```python
from build123d import *

# Parameters (mm, degrees)
SKETCH1_W                = 14.986
SKETCH1_H                = 10.16
BOSS_EXTRUDE1_DEPTH      = 3.175
M3_CLEARANCE_HOLE1_D     = 3.4
M3_CLEARANCE_HOLE1_DEPTH = 10
M3_CLEARANCE_HOLE1_TIP   = 1.021463052
SKETCH4_R                = 0.396875
CUT_EXTRUDE1_DEPTH       = 19.38168711


with BuildPart() as part:
    # Sketch1 → Boss-Extrude1 (new body)
    with BuildSketch(Plane.XY):
        with Locations((7.493, 5.08)):
            Rectangle(SKETCH1_W, SKETCH1_H)
    extrude(amount=BOSS_EXTRUDE1_DEPTH)

    # M3 Clearance Hole1
    with Locations(Plane.XY.offset(3.175)):
        with Locations((10.9982, 5.08), (3.9878, 5.08)):
            Hole(M3_CLEARANCE_HOLE1_D / 2, depth=M3_CLEARANCE_HOLE1_DEPTH)
            with Locations((0, 0, -(M3_CLEARANCE_HOLE1_DEPTH + M3_CLEARANCE_HOLE1_TIP / 2))):  # 118° drill point
                Cone(0, M3_CLEARANCE_HOLE1_D / 2, M3_CLEARANCE_HOLE1_TIP, mode=Mode.SUBTRACT)

    # Sketch4 → Cut-Extrude1 (cut, through all)
    with BuildSketch(Plane.XY.offset(3.175)):
        with Locations((7.493, 5.08)):
            Circle(SKETCH4_R)
    extrude(amount=-CUT_EXTRUDE1_DEPTH, mode=Mode.SUBTRACT)


solid = part.part
```
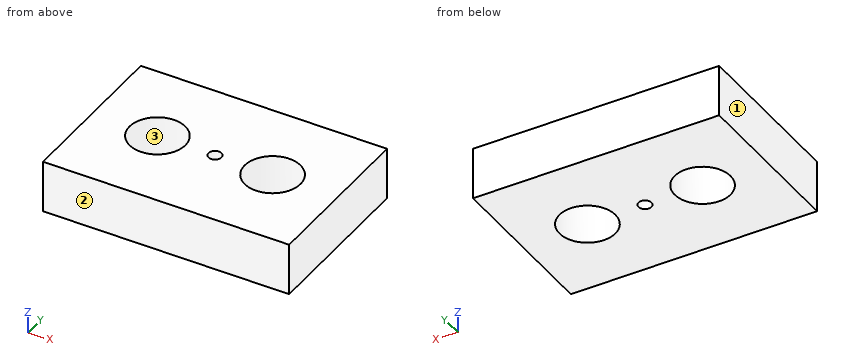
The model under review builds one solid part; all positions refer to its coordinate system, in mm. Face numbers are marked on the shaded views. Give positions to 0.01 mm unless a question says otherwise; leave off trailing zeros. Write each loop counter-clockwise with the first axis right and the second up, starting at its lowest first coordinate (ties: lowest second). Pieces come first, ordered by that corner, then holes. Notation, with made-up numbers: (11, 77.25) - (35, 77.25) arc R22 ccw to (35, 97.25) - close; hole circle Ø11 at (72, -5). An arc over 180 degrees is marked (long way). Answer in a Markdown table with one row per item. Add a question column.
1. We need section A-A on y = 5.08. Write out the cut boundary in (x, z) (3 decimals).
2. Draft analysis for pull direction X (two halves, no side actions). For the marked faces 1, 2 and 3, state which applies: +X half, -X half, draft (parallel to the pull), parting line (faces both ways), or undercut.
3. Wall thickness on line 1 along X through (y, z) = (4.75, 2.3); line 2 along Y through (x, z) = (7.5, 2.8); line 3 along X through (y, z) = (4, 0.55): over which ranges is each line inside the solid? List them lowest first. Write a range as [from, to].
4. We need section B-B on x = 9.5. Write out the cut boundary in (y, z) (3 decimals).
5. We need section C-C on z = 0.7. Write out the cut boundary in (x, y).
Ans:
| question | item | result |
|---|---|---|
| 1 | outline | (0, 0) - (2.288, 0) - (2.288, 3.175) - (0, 3.175) - close; (5.688, 0) - (7.096, 0) - (7.096, 3.175) - (5.688, 3.175) - close; (7.89, 0) - (9.298, 0) - (9.298, 3.175) - (7.89, 3.175) - close; (12.698, 0) - (14.986, 0) - (14.986, 3.175) - (12.698, 3.175) - close |
| 2 | face 1 | -X half |
| 2 | face 2 | draft |
| 2 | face 3 | undercut |
| 3 | line 1 | x = [0, 2.32], [5.66, 7.27], [7.71, 9.33], [12.67, 14.99] |
| 3 | line 2 | y = [0, 4.68], [5.48, 10.16] |
| 3 | line 3 | x = [0, 2.67], [5.3, 9.69], [12.31, 14.99] |
| 4 | outline | (0, 0) - (4.277, 0) - (4.277, 3.175) - (0, 3.175) - close; (5.883, 0) - (10.16, 0) - (10.16, 3.175) - (5.883, 3.175) - close |
| 5 | outline | (0, 0) - (14.99, 0) - (14.99, 10.16) - (0, 10.16) - close; hole circle Ø3.4 at (3.99, 5.08); hole circle Ø0.79 at (7.49, 5.08); hole circle Ø3.4 at (11, 5.08) |
